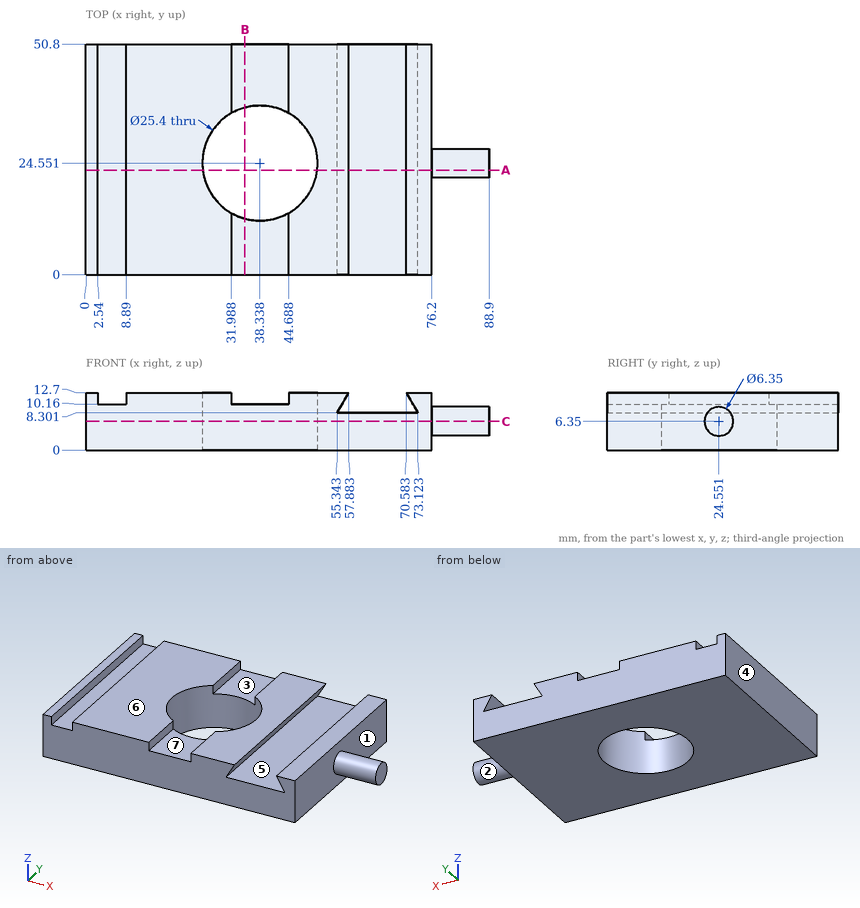
Geometry check sheet. Reference: drawing and pictorial views, mm from the part's lowest x, y, z. A direction names the side the tool comes from. Coordinates: 2 decimals unless noted, no trailing zeros. Loops run counter-clockwise (first coordinate to the right, second up) from the corner with the lowest first, then second, coordinate; pieces in that order, holes last.
1) Access from +Z, -Z, +X, -X, +Y, -Y to the whole of each face (thin tool, end or side, straight path). Record for the marked faces 5, 6 and 7.
2) Gauge pin test, flat ends, axial feed: pin 1 (5 mm diameter, centred on y = 33.5, z = 8, fed in from +X); pin 2 (5.5 mm diameter, centred on x = 67.5, y = 36.5, fed in from +Z); pin 3 (3 mm diameter, centred on x = 6, y = 27.5, fed in from +Z). Record the tip position at first contact, or that the pin passes through.
3) Material ranges on probe 1 along X at (y, z) = (19.5, 9.5) (1 decimal); probe 2 along X at (y, z) = (16, 10.75); probe 3 along X at (y, z) = (48, 9), recorded low to high.
4) Sectioned sample at B-B (x = 35). Record the boundary of the cut face in (y, z) (1 decimal), and give its area (3 significant figures).
5) Sectioned sample at C-C (z = 6.35). Record the boundary of the cut face in (x, y).
6) Sectioned sample at A-A (y = 23). Record the boundary of the cut face in (x, z), and give its area (3 significant figures).
7) Release check for a two-part mould opening along X. For the marked faces 1, 2, 3 and 4 record: released by +X, released by -X, zero draft, split by the parting line, or undercut.
Check sheet entries:
1. face 5: +Y, -Y
1. face 6: +Z, +X, -X, +Y, -Y
1. face 7: +Z, +Y, -Y
2. pin 1: stops at x = 76.2
2. pin 2: stops at z = 8.3
2. pin 3: stops at z = 10.16
3. probe 1: x = 0 to 26.7, 50 to 56, 72.4 to 76.2
3. probe 2: x = 0 to 2.54, 8.89 to 28.95, 47.73 to 56.76, 71.71 to 76.2
3. probe 3: x = 0 to 55.75, 72.72 to 76.2
4. outline: (0, 0) - (12.3, 0) - (12.3, 10.2) - (0, 10.2) - close; (36.8, 0) - (50.8, 0) - (50.8, 10.2) - (36.8, 10.2) - close
4. area: 267 mm2
5. outline: (0, 0) - (76.2, 0) - (76.2, 21.38) - (88.9, 21.38) - (88.9, 27.73) - (76.2, 27.73) - (76.2, 50.8) - (0, 50.8) - close; hole circle Ø25.4 at (38.34, 24.55)
6. outline: (0, 0) - (25.73, 0) - (25.73, 12.7) - (8.89, 12.7) - (8.89, 10.16) - (2.54, 10.16) - (2.54, 12.7) - (0, 12.7) - close; (50.94, 0) - (76.2, 0) - (76.2, 3.58) - (88.9, 3.58) - (88.9, 9.12) - (76.2, 9.12) - (76.2, 12.7) - (70.58, 12.7) - (73.12, 8.3) - (55.34, 8.3) - (57.88, 12.7) - (50.94, 12.7) - close
6. area: 635 mm2
7. face 1: released by +X
7. face 2: zero draft
7. face 3: undercut
7. face 4: released by -X
